from build123d import *

# Parameters (mm, degrees)
BOSS_EXTRUDE1_DEPTH = 2
FILLET1_R           = 5
SKETCH2_R           = 1.6
CUT_EXTRUDE1_DEPTH  = 38.553295461
MOVE_FACE1_BY       = 0.5
MOVE_FACE1_2_BY     = 0.5
MOVE_FACE1_3_BY     = 0.5
MOVE_FACE1_4_BY     = 0.5
MOVE_FACE1_5_BY     = 0.5
MOVE_FACE1_6_BY     = 0.5
MOVE_FACE1_7_BY     = 0.5
MOVE_FACE1_8_BY     = 0.5
MOVE_FACE1_9_BY     = 0.5
MOVE_FACE1_10_BY    = 0.5
MOVE_FACE1_11_BY    = 0.5
MOVE_FACE1_12_BY    = 0.5
MOVE_FACE1_13_BY    = 0.5
MOVE_FACE1_14_BY    = 0.5
MOVE_FACE1_15_BY    = 0.5
MOVE_FACE1_16_BY    = 0.5
DRAFT1_ANGLE        = -3
BOSS_EXTRUDE3_DEPTH = 1
BOSS_EXTRUDE3_DRAFT = 3
FILLET3_R           = 0.5
CUT_EXTRUDE2_DEPTH  = 0.2
CUT_EXTRUDE2_DRAFT  = -3


with BuildPart() as part:
    # Sketch1 → Boss-Extrude1 (new body)
    with BuildSketch(Plane.XY):
        Polygon((-7.5, 30), (7.5, 30), (7.5, 0), (22.5, 0), (22.5, -15), (-22.5, -15), (-22.5, 0), (-7.5, 0), align=None)
    extrude(amount=BOSS_EXTRUDE1_DEPTH)

    # Fillet1
    fillet1_edges = [part.edges().sort_by_distance(p)[0] for p in [
        (-7.5, 30, 1),
        (7.5, 30, 1),
        (7.5, 0, 1),
        (22.5, 0, 1),
        (22.5, -15, 1),
        (-22.5, -15, 1),
        (-22.5, 0, 1),
        (-7.5, 0, 1),
    ]]
    fillet(fillet1_edges, radius=FILLET1_R)

    # Sketch2 → Cut-Extrude1 (cut, through all)
    with BuildSketch(Plane.XY.offset(2)):
        with Locations((-15, -7.5)):
            Circle(SKETCH2_R)
        with Locations((0, -7.5)):
            Circle(SKETCH2_R)
        with Locations((15, -7.5)):
            Circle(SKETCH2_R)
        with Locations((0, 22.5)):
            Circle(SKETCH2_R)
        with Locations((0, 7.5)):
            Circle(SKETCH2_R)
    extrude(amount=-CUT_EXTRUDE1_DEPTH, mode=Mode.SUBTRACT)

    # Move Face1: a curved face moved inward by 0.5
    add(Solid.thicken(part.faces().sort_by_distance((-8.964466094, 1.464466094, 1))[0], -MOVE_FACE1_BY), mode=Mode.SUBTRACT)

    # Move Face1 2: a face moved inward by 0.5
    extrude(part.faces().sort_by_distance((-15, 0, 1))[0], amount=MOVE_FACE1_2_BY, dir=(0, -1, 0), mode=Mode.SUBTRACT)

    # Move Face1 3: a curved face moved inward by 0.5
    add(Solid.thicken(part.faces().sort_by_distance((-21.035533906, -1.464466094, 1))[0], -MOVE_FACE1_3_BY), mode=Mode.SUBTRACT)

    # Move Face1 4: a face moved inward by 0.5
    extrude(part.faces().sort_by_distance((-22.5, -7.5, 1))[0], amount=MOVE_FACE1_4_BY, dir=(1, 0, 0), mode=Mode.SUBTRACT)

    # Move Face1 5: a curved face moved inward by 0.5
    add(Solid.thicken(part.faces().sort_by_distance((-21.035533906, -13.535533906, 1))[0], -MOVE_FACE1_5_BY), mode=Mode.SUBTRACT)

    # Move Face1 6: a face moved inward by 0.5
    extrude(part.faces().sort_by_distance((0, -15, 1))[0], amount=MOVE_FACE1_6_BY, dir=(0, 1, 0), mode=Mode.SUBTRACT)

    # Move Face1 7: a curved face moved inward by 0.5
    add(Solid.thicken(part.faces().sort_by_distance((21.035533906, -13.535533906, 1))[0], -MOVE_FACE1_7_BY), mode=Mode.SUBTRACT)

    # Move Face1 8: a face moved inward by 0.5
    extrude(part.faces().sort_by_distance((22.5, -7.5, 1))[0], amount=MOVE_FACE1_8_BY, dir=(-1, 0, 0), mode=Mode.SUBTRACT)

    # Move Face1 9: a curved face moved inward by 0.5
    add(Solid.thicken(part.faces().sort_by_distance((21.035533906, -1.464466094, 1))[0], -MOVE_FACE1_9_BY), mode=Mode.SUBTRACT)

    # Move Face1 10: a face moved inward by 0.5
    extrude(part.faces().sort_by_distance((15, 0, 1))[0], amount=MOVE_FACE1_10_BY, dir=(0, -1, 0), mode=Mode.SUBTRACT)

    # Move Face1 11: a curved face moved inward by 0.5
    add(Solid.thicken(part.faces().sort_by_distance((8.964466094, 1.464466094, 1))[0], -MOVE_FACE1_11_BY), mode=Mode.SUBTRACT)

    # Move Face1 12: a face moved inward by 0.5
    extrude(part.faces().sort_by_distance((7.5, 15, 1))[0], amount=MOVE_FACE1_12_BY, dir=(-1, 0, 0), mode=Mode.SUBTRACT)

    # Move Face1 13: a curved face moved inward by 0.5
    add(Solid.thicken(part.faces().sort_by_distance((6.035533906, 28.535533906, 1))[0], -MOVE_FACE1_13_BY), mode=Mode.SUBTRACT)

    # Move Face1 14: a face moved inward by 0.5
    extrude(part.faces().sort_by_distance((0, 30, 1))[0], amount=MOVE_FACE1_14_BY, dir=(0, -1, 0), mode=Mode.SUBTRACT)

    # Move Face1 15: a curved face moved inward by 0.5
    add(Solid.thicken(part.faces().sort_by_distance((-6.035533906, 28.535533906, 1))[0], -MOVE_FACE1_15_BY), mode=Mode.SUBTRACT)

    # Move Face1 16: a face moved inward by 0.5
    extrude(part.faces().sort_by_distance((-7.5, 15, 1))[0], amount=MOVE_FACE1_16_BY, dir=(1, 0, 0), mode=Mode.SUBTRACT)

    # Draft1
    draft1_faces = [part.faces().sort_by_distance(p)[0] for p in [
        (13.4, -7.5, 1),
        (-1.6, 22.5, 1),
        (-1.6, 7.5, 1),
        (-1.6, -7.5, 1),
        (-16.6, -7.5, 1),
        (-20.681980515, -1.818019485, 1),
        (-22, -7.5, 1),
        (-20.681980515, -13.181980515, 1),
        (0, -14.5, 1),
        (20.681980515, -13.181980515, 1),
        (22, -7.5, 1),
        (20.681980515, -1.818019485, 1),
        (15, -0.5, 1),
        (8.610912703, 1.110912703, 1),
        (7, 15, 1),
        (5.681980515, 28.181980515, 1),
        (0, 29.5, 1),
        (-5.681980515, 28.181980515, 1),
        (-7, 15, 1),
        (-8.610912703, 1.110912703, 1),
        (-15, -0.5, 1),
    ]]
    draft(draft1_faces, Plane(origin=(0, 0, 0), x_dir=(-1, 0, 0), z_dir=(0, 0, -1)), DRAFT1_ANGLE)


with BuildPart() as boss_extrude3_tool:
    # Sketch4 → Boss-Extrude3 (with draft: the straight prism first)
    with BuildSketch(Plane.XY.offset(2)):
        with BuildLine():
            Line((-17.5, -14.395184441), (17.5, -14.395184441))
            ThreePointArc((17.5, -14.395184441), (20.607864723, -13.107864723), (21.895184441, -10))
            Line((21.895184441, -10), (21.895184441, -5))
            ThreePointArc((21.895184441, -5), (20.607864723, -1.892135277), (17.5, -0.604815559))
            Line((17.5, -0.604815559), (12.5, -0.604815559))
            ThreePointArc((12.5, -0.604815559), (8.536796911, 1.036796911), (6.895184441, 5))
            Line((6.895184441, 5), (6.895184441, 25))
            ThreePointArc((6.895184441, 25), (5.607864723, 28.107864723), (2.5, 29.395184441))
            Line((2.5, 29.395184441), (-2.5, 29.395184441))
            ThreePointArc((-2.5, 29.395184441), (-5.607864723, 28.107864723), (-6.895184441, 25))
            Line((-6.895184441, 25), (-6.895184441, 5))
            ThreePointArc((-6.895184441, 5), (-8.536796911, 1.036796911), (-12.5, -0.604815559))
            Line((-12.5, -0.604815559), (-17.5, -0.604815559))
            ThreePointArc((-17.5, -0.604815559), (-20.607864723, -1.892135277), (-21.895184441, -5))
            Line((-21.895184441, -5), (-21.895184441, -10))
            ThreePointArc((-21.895184441, -10), (-20.607864723, -13.107864723), (-17.5, -14.395184441))
        make_face()
        with BuildLine():
            Line((-17.5, -12.921388331), (17.5, -12.921388331))
            ThreePointArc((17.5, -12.921388331), (19.565733499, -12.065733499), (20.421388331, -10))
            Line((20.421388331, -10), (20.421388331, -5))
            ThreePointArc((20.421388331, -5), (19.565733499, -2.934266501), (17.5, -2.078611669))
            Line((17.5, -2.078611669), (12.5, -2.078611669))
            ThreePointArc((12.5, -2.078611669), (7.494665688, -0.005334312), (5.421388331, 5))
            Line((5.421388331, 5), (5.421388331, 25))
            ThreePointArc((5.421388331, 25), (4.565733499, 27.065733499), (2.5, 27.921388331))
            Line((2.5, 27.921388331), (-2.5, 27.921388331))
            ThreePointArc((-2.5, 27.921388331), (-4.565733499, 27.065733499), (-5.421388331, 25))
            Line((-5.421388331, 25), (-5.421388331, 5))
            ThreePointArc((-5.421388331, 5), (-7.494665688, -0.005334312), (-12.5, -2.078611669))
            Line((-12.5, -2.078611669), (-17.5, -2.078611669))
            ThreePointArc((-17.5, -2.078611669), (-19.565733499, -2.934266501), (-20.421388331, -5))
            Line((-20.421388331, -5), (-20.421388331, -10))
            ThreePointArc((-20.421388331, -10), (-19.565733499, -12.065733499), (-17.5, -12.921388331))
        make_face(mode=Mode.SUBTRACT)
    extrude(amount=BOSS_EXTRUDE3_DEPTH)
    # Boss-Extrude3: the draft: its side faces are tilted about the plane it starts from
    boss_extrude3_sides = [boss_extrude3_tool.faces().sort_by_distance(p)[0] for p in [
        (-20.607864723, -1.892135277, 2.5),
        (-21.895184441, -7.5, 2.5),
        (-20.607864723, -13.107864723, 2.5),
        (0, -14.395184441, 2.5),
        (20.607864723, -13.107864723, 2.5),
        (21.895184441, -7.5, 2.5),
        (20.607864723, -1.892135277, 2.5),
        (15, -0.604815559, 2.5),
        (8.536796911, 1.036796911, 2.5),
        (6.895184441, 15, 2.5),
        (5.607864723, 28.107864723, 2.5),
        (0, 29.395184441, 2.5),
        (-5.607864723, 28.107864723, 2.5),
        (-6.895184441, 15, 2.5),
        (-8.536796911, 1.036796911, 2.5),
        (-15, -0.604815559, 2.5),
        (-15, -2.078611669, 2.5),
        (-7.494665688, -0.005334312, 2.5),
        (-5.421388331, 15, 2.5),
        (-4.565733499, 27.065733499, 2.5),
        (0, 27.921388331, 2.5),
        (4.565733499, 27.065733499, 2.5),
        (5.421388331, 15, 2.5),
        (7.494665688, -0.005334312, 2.5),
        (15, -2.078611669, 2.5),
        (19.565733499, -2.934266501, 2.5),
        (20.421388331, -7.5, 2.5),
        (19.565733499, -12.065733499, 2.5),
        (0, -12.921388331, 2.5),
        (-19.565733499, -12.065733499, 2.5),
        (-20.421388331, -7.5, 2.5),
        (-19.565733499, -2.934266501, 2.5),
    ]]
    draft(boss_extrude3_sides, Plane.XY.offset(2), BOSS_EXTRUDE3_DRAFT)


with BuildPart() as part_1:
    add(part.part)

    # Boss-Extrude3: add boss_extrude3_tool
    add(boss_extrude3_tool.part)

    # Fillet3
    fillet3_edges = [part_1.edges().sort_by_distance(p)[0] for p in [
        (-20.570806827, -13.070806827, 3),
        (0, -14.342776662, 3),
        (20.570806827, -13.070806827, 3),
        (21.842776662, -7.5, 3),
        (20.570806827, -1.929193173, 3),
        (15, -0.657223338, 3),
        (8.499739015, 0.999739015, 3),
        (6.842776662, 15, 3),
        (5.570806827, 28.070806827, 3),
        (0, 29.342776662, 3),
        (-5.570806827, 28.070806827, 3),
        (-6.842776662, 15, 3),
        (-8.499739015, 0.999739015, 3),
        (-15, -0.657223338, 3),
        (-20.570806827, -1.929193173, 3),
        (-21.842776662, -7.5, 3),
        (-19.602791396, -12.102791396, 3),
        (0, -12.97379611, 3),
        (19.602791396, -12.102791396, 3),
        (20.47379611, -7.5, 3),
        (19.602791396, -2.897208604, 3),
        (15, -2.02620389, 3),
        (7.531723584, 0.031723584, 3),
        (5.47379611, 15, 3),
        (4.602791396, 27.102791396, 3),
        (0, 27.97379611, 3),
        (-4.602791396, 27.102791396, 3),
        (-5.47379611, 15, 3),
        (-7.531723584, 0.031723584, 3),
        (-15, -2.02620389, 3),
        (-19.602791396, -2.897208604, 3),
        (-20.47379611, -7.5, 3),
    ]]
    fillet(fillet3_edges, radius=FILLET3_R)


with BuildPart() as cut_extrude2_tool:
    # Sketch5 → Cut-Extrude2 (with draft: the straight prism first)
    with BuildSketch(Plane(origin=(0, 0, 0), x_dir=(-1, 0, 0), z_dir=(0, 0, -1))):
        with BuildLine():
            Line((-14.5, -13.8), (14.5, -13.8))
            ThreePointArc((14.5, -13.8), (14.853553391, -13.653553391), (15, -13.3))
            Line((15, -13.3), (15, -10.3))
            ThreePointArc((15, -10.3), (14.853553391, -9.946446609), (14.5, -9.8))
            Line((14.5, -9.8), (-14.5, -9.8))
            ThreePointArc((-14.5, -9.8), (-14.853553391, -9.946446609), (-15, -10.3))
            Line((-15, -10.3), (-15, -13.3))
            ThreePointArc((-15, -13.3), (-14.853553391, -13.653553391), (-14.5, -13.8))
        make_face()
    extrude(amount=-CUT_EXTRUDE2_DEPTH)
    # Cut-Extrude2: the draft: its side faces are tilted about the plane it starts from
    cut_extrude2_sides = [cut_extrude2_tool.faces().sort_by_distance(p)[0] for p in [
        (0, -13.8, 0.1),
        (-14.853553391, -13.653553391, 0.1),
        (-15, -11.8, 0.1),
        (-14.853553391, -9.946446609, 0.1),
        (0, -9.8, 0.1),
        (14.853553391, -9.946446609, 0.1),
        (15, -11.8, 0.1),
        (14.853553391, -13.653553391, 0.1),
    ]]
    draft(cut_extrude2_sides, Plane(origin=(0, 0, 0), x_dir=(-1, 0, 0), z_dir=(0, 0, -1)), CUT_EXTRUDE2_DRAFT)


with BuildPart() as part_2:
    add(part_1.part)

    # Cut-Extrude2: cut by cut_extrude2_tool
    add(cut_extrude2_tool.part, mode=Mode.SUBTRACT)


solid = part_2.part
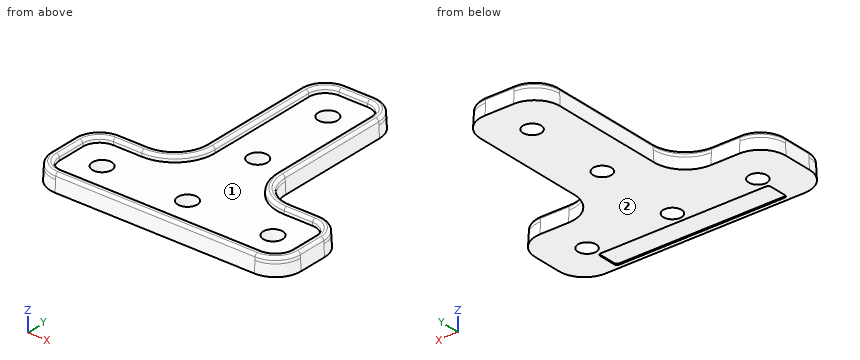
Read the model definition and answer for the solid it produces. Units are mm, in the model's axes. Face numbers are marked on the shaded views. Round coordinates to 2 decimals unless told otherwise and drop trailing zeros. Write each loop counter-clockwise with the first axis right and the second up, starting at its lowest first coordinate (ties: lowest second). Pieces come first, ordered by that corner, then holes. Notation, with made-up numbers: M 64.25,-4.75 L 114.25,-4.75 A19 cw 114.25,4.25 Z; hole C 86,68.25 d4. An arc over 180 degrees is marked long. Use a Markdown table: item, result.
1) The part is cut by section D-D (z = 1.4). Write down the section's boundary in (x, y), plus the area to 3 significant figures.
Answers follow:
| item | result |
|---|---|
| outline | M -21.93,-10 A4.43 ccw -17.5,-14.43 L 17.5,-14.43 A4.43 ccw 21.93,-10 L 21.93,-5 A4.43 ccw 17.5,-0.57 L 12.5,-0.57 A5.57 cw 6.93,5 L 6.93,25 A4.43 ccw 2.5,29.43 L -2.5,29.43 A4.43 ccw -6.93,25 L -6.93,5 A5.57 cw -12.5,-0.57 L -17.5,-0.57 A4.43 ccw -21.93,-5 Z; hole C -15,-7.5 d3.35; hole C 0,-7.5 d3.35; hole C 0,7.5 d3.35; hole C 0,22.5 d3.35; hole C 15,-7.5 d3.35 |
| area | 967 mm2 |
2) For a pull along X with two mould halves and no side action, classify the marked faces 1 and 2 as pulls with the +X half, pulls with the -X half, needs draft (parallel to the pull), parting line crosses it, or undercut.
Answers follow:
| item | result |
|---|---|
| face 1 | undercut |
| face 2 | needs draft |
3) The part is cut by section B-B (x = 0). Write down the section's boundary in (y, z).
Answers follow:
| item | result |
|---|---|
| outline | M -14.5,0 L -13.8,0 L -13.79,0.2 L -9.81,0.2 L -9.8,0 L -9.1,0 L -9.2,2 L -12.92,2 L -12.95,2.53 A0.5 ccw -13.45,3 L -13.87,3 A0.5 ccw -14.37,2.53 Z; M -5.9,0 L 5.9,0 L 5.8,2 L -5.8,2 Z; M 9.1,0 L 20.9,0 L 20.8,2 L 9.2,2 Z; M 24.1,0 L 29.5,0 L 29.37,2.53 A0.5 ccw 28.87,3 L 28.45,3 A0.5 ccw 27.95,2.53 L 27.92,2 L 24.2,2 Z |
4) Straight lines are drawn through the part: line 1 along Y through (x, z) = (-15, 1.85); line 2 along X through (y, z) = (14.5, 2.5); line 3 along Y through (x, z) = (-15, 2.6). For each, find the intervals that lie inside material, in ascending order. Write a range as [from, to].
Answers follow:
| item | result |
|---|---|
| line 1 | y = [-14.4, -9.2], [-5.8, -0.6] |
| line 2 | x = [-6.87, -5.45], [5.45, 6.87] |
| line 3 | y = [-14.36, -12.96], [-2.04, -0.64] |
5) The part is cut by section C-C (y = -7.5). Write down the section's boundary in (x, z).
Answers follow:
| item | result |
|---|---|
| outline | M -22,0 L -16.6,0 L -16.7,2 L -20.42,2 L -20.45,2.53 A0.5 ccw -20.95,3 L -21.37,3 A0.5 ccw -21.87,2.53 Z; M -13.4,0 L -1.6,0 L -1.7,2 L -13.3,2 Z; M 1.6,0 L 13.4,0 L 13.3,2 L 1.7,2 Z; M 16.6,0 L 22,0 L 21.87,2.53 A0.5 ccw 21.37,3 L 20.95,3 A0.5 ccw 20.45,2.53 L 20.42,2 L 16.7,2 Z |
6) A flat-ended cylindrical pin translates along its axis: pin 1 (1.5 mm diameter, centred on x = 1.5, y = 5.5, fed in from +Z). Find the tip coordinate at first contact, or state that the pin passes through.
Answers follow:
| item | result |
|---|---|
| pin 1 | stops at z = 2 |
7) The part is cut by section A-A (y = 22.5). Write down the section's boundary in (x, z).
Answers follow:
| item | result |
|---|---|
| outline | M -7,0 L -1.6,0 L -1.7,2 L -5.42,2 L -5.45,2.53 A0.5 ccw -5.95,3 L -6.37,3 A0.5 ccw -6.87,2.53 Z; M 1.6,0 L 7,0 L 6.87,2.53 A0.5 ccw 6.37,3 L 5.95,3 A0.5 ccw 5.45,2.53 L 5.42,2 L 1.7,2 Z |
